Check sheet for the modelled part. Datum: model origin and axes. Units: mm. Give positions to 0.01 mm unless a question says otherwise; leave off trailing zeros. Order: outer loops, then holes, each group sorted by start corner. A loop starts at its lowest first (then second) coordinate and runs counter-clockwise, first axis right, second up. Notation, with made-up numbers: (-3.5, 77) - (47.5, 77) arc R21 ccw to (47.5, 86) - close; hole circle Ø4 at (7, -39.75). An arc over 180 degrees is marked (long way). Answer in a Markdown table with one row per item.
from build123d import *

# Parameters (mm, degrees)
SKETCH1_R           = 2
BOSS_EXTRUDE1_DEPTH = 32
SKETCH2_R           = 7.5
CUT_EXTRUDE1_DEPTH  = 25


with BuildPart() as part:
    # Sketch1 → Boss-Extrude1 (new body)
    with BuildSketch(Plane(origin=(0, 0, 0), x_dir=(1, 0, 0), z_dir=(0, 1, 0))):
        with BuildLine():
            Line((-13.772808121, -0.151299578), (-14, 0))
            ThreePointArc((-14, 0), (-21.863703305, 1.03527618), (-14.535898385, -2))
            add(Edge.make_bspline(
                [(-14.535898385, -2), (0, -8), (14.535898385, -2)],
                knots=[0, 0, 0, 1, 1, 1], degree=2))
            ThreePointArc((14.535898385, -2), (21.863703305, 1.03527618), (14, 0))
            Line((14, 0), (13.772808121, -0.151299578))
            add(Edge.make_bspline(
                [(-13.772808121, -0.151299578), (-13.200157242, -0.38767336), (-12.03616489, -0.83828907), (-9.734990662, -1.609651667), (-6.861177209, -2.35105477), (-3.427724467, -2.882094844), (0, -3.058952578), (3.427724467, -2.882094844), (6.861177209, -2.35105477), (9.734990662, -1.609651667), (12.03616489, -0.83828907), (13.200157242, -0.38767336), (13.772808121, -0.151299578)],
                knots=[0, 0, 0, 0, 0.0625, 0.125, 0.25, 0.375, 0.5, 0.625, 0.75, 0.875, 0.9375, 1, 1, 1, 1], degree=3))
        make_face()
        with Locations(Location((-18, 0, 0), (0, 0, 270))):
            Circle(SKETCH1_R, mode=Mode.SUBTRACT)
        with Locations(Location((18, 0, 0), (0, 0, 270))):
            Circle(SKETCH1_R, mode=Mode.SUBTRACT)
    extrude(amount=BOSS_EXTRUDE1_DEPTH)

    # Sketch2 → Cut-Extrude1 (cut)
    with BuildSketch(Plane.XY):
        with Locations(Location((0, 16, 0), (0, 0, 180))):
            Circle(SKETCH2_R)
    extrude(amount=CUT_EXTRUDE1_DEPTH, mode=Mode.SUBTRACT)


solid = part.part
(1) Gauge pin test, flat ends, axial feed: P1, Ø4, axis at x = -2.5, y = 8, coming from the -Z side; P2, Ø6, axis at x = -17.5, y = 29, coming from the +Z side; P3, Ø3, axis at x = -1, y = 27, coming from the -Z side. Record the tip position at first contact, or that the pin passes through.
Geometry says:
| item | result |
|---|---|
| P1 | z = 2.7 |
| P2 | z = 4 |
| P3 | z = 2.91 |
(2) Thickness scan on L1, parallel to X at y = 28.5, z = -0.25; L2, parallel to X at y = 6, z = -3; L3, parallel to Z at x = 19.5, y = 22. Record the ranges inside material, lowest first.
Geometry says:
| item | result |
|---|---|
| L1 | -21.99 to -19.98, -16.02 to -14.01, 14.01 to 16.02, 19.98 to 21.99 |
| L2 | -20.65 to -15.35, 15.35 to 20.65 |
| L3 | -3.71 to -1.32, 1.32 to 3.71 |
(3) Cross-section at A-A, the plane x = 18. Record the cut outline in (y, z).
Geometry says:
| item | result |
|---|---|
| outline | (0, -4) - (32, -4) - (32, -2) - (0, -2) - close; (0, 2) - (32, 2) - (32, 4) - (0, 4) - close |
(4) Cross-section at C-C, the plane y = 4. Give the number of separate pieces and of enclosed holes in the cut face, then the cut area to 3 significant figures.
Geometry says:
| item | result |
|---|---|
| separate pieces | 1 |
| enclosed holes | 2 |
| area | 134 mm² |
(5) Cross-section at B-B, the plane z = -2.75. Record the cut outline in (x, y).
Geometry says:
| item | result |
|---|---|
| outline | (-20.9, 0) - (-15.1, 0) - (-15.1, 32) - (-20.9, 32) - close; (15.1, 0) - (20.9, 0) - (20.9, 32) - (15.1, 32) - close |
(6) Mould release check, pull along Y, two halves, no side actions. Record for faces 1 (the cylindrical face through (21.9, 15.78, -0.88)), 2 (the flat face through (-1.7, 0, 3.3)), 3 (the cylindrical face through (-6.93, 18.87, 3.56)): pulls with the +Y half, pulls with the -Y half, needs draft (parallel to the pull), parting line crosses it, or undercut.
Geometry says:
| item | result |
|---|---|
| face 1 | needs draft |
| face 2 | pulls with the -Y half |
| face 3 | undercut |
